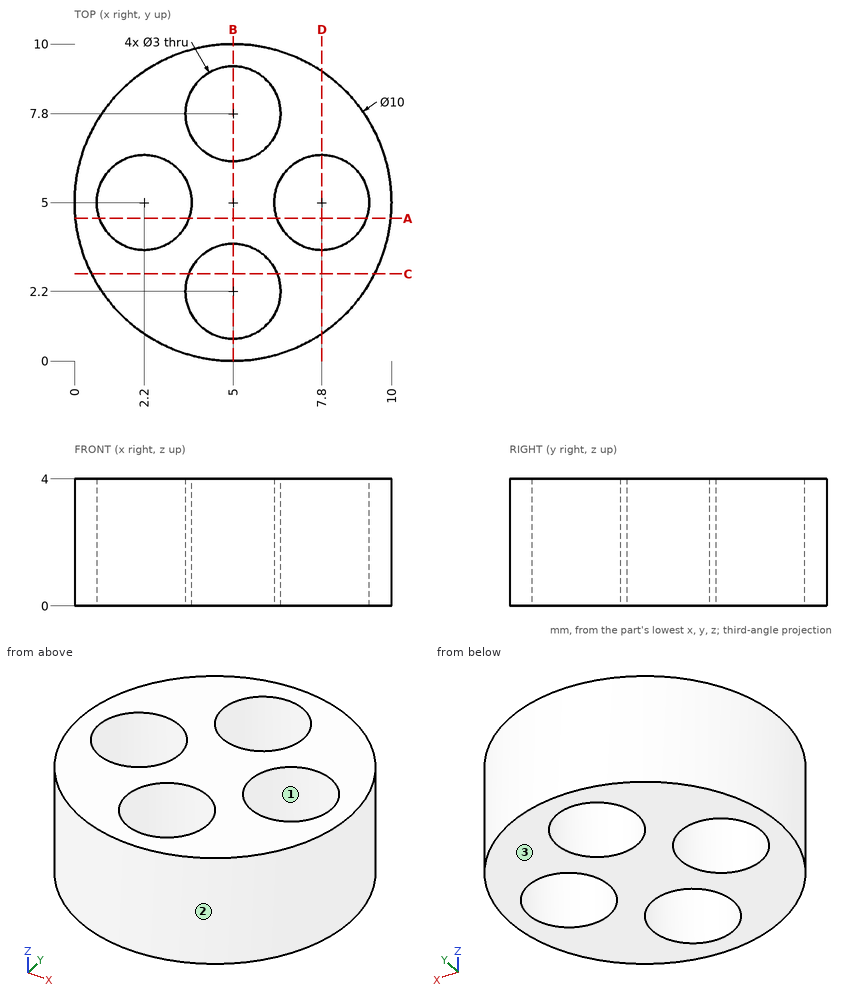
For this review, use the dimensioned drawing (mm, ordinates from the lowest corner) and the shaded views. Coordinates: 2 decimals unless noted, no trailing zeros. Order: outer loops, then holes, each group sorted by start corner. A loop starts at its lowest first (then second) coordinate and runs counter-clockwise, first axis right, second up. Notation, with made-up numbers: (75.25, 42.25) - (116.25, 42.25) arc R9 ccw to (116.25, 54.25) - close; hole circle Ø9 at (22, 51.5). An arc over 180 degrees is marked (long way). Answer as a JSON object with one key per item and string values. Group by question number.
1. We need section D-D on x = 7.8. State the section outline as (y, z) points.
2. We need section C-C on y = 2.75. State the section outline as (x, z) points, then the cut area to 3 significant figures.
3. For probe 1 along X at (y, z) = (5, 3.6); probe 2 along Y at (x, z) = (6.25, 2); probe 3 along X at (y, z) = (1, 3.5), list the stretches that pass through material, from the lowest coordinate up.
4. Clearance check with flat-ended pins moving along their axes: P1, Ø1.5, axis at y = 6, z = 3.5, coming from the -X side; P2, Ø2.5, axis at x = 7.8, y = 5, coming from the +Z side; P3, Ø1.5, axis at y = 7, z = 3.5, coming from the +X side. State where each tip first meets the part, or that it passes through.
5. We need section A-A on y = 4.5. State the section outline as (x, z) points.
6. We need section B-B on x = 5. State the section outline as (y, z) points.
7. The part is to be moulded in two halves that separate along Y. For the marked faces 1, 2 and 3, say which applies: pulls with the +Y half, pulls with the -Y half, needs draft (parallel to the pull), parting line crosses it, or undercut.
Final values:
{
 "1": {"outline": "(0.86, 0) - (3.5, 0) - (3.5, 4) - (0.86, 4) - close; (6.5, 0) - (9.14, 0) - (9.14, 4) - (6.5, 4) - close"},
 "2": {"outline": "(0.53, 0) - (3.6, 0) - (3.6, 4) - (0.53, 4) - close; (6.4, 0) - (9.47, 0) - (9.47, 4) - (6.4, 4) - close", "area": "24.6 mm²"},
 "3": {"probe 1": "0 to 0.7, 3.7 to 6.3, 9.3 to 10", "probe 2": "0.16 to 1.37, 3.03 to 6.97, 8.63 to 9.84", "probe 3": "2 to 4.1, 5.9 to 8"},
 "4": {"P1": "x = 0.01", "P2": "through", "P3": "x = 9.84"},
 "5": {"outline": "(0.03, 0) - (0.79, 0) - (0.79, 4) - (0.03, 4) - close; (3.61, 0) - (6.39, 0) - (6.39, 4) - (3.61, 4) - close; (9.21, 0) - (9.97, 0) - (9.97, 4) - (9.21, 4) - close"},
 "6": {"outline": "(0, 0) - (0.7, 0) - (0.7, 4) - (0, 4) - close; (3.7, 0) - (6.3, 0) - (6.3, 4) - (3.7, 4) - close; (9.3, 0) - (10, 0) - (10, 4) - (9.3, 4) - close"},
 "7": {"face 1": "undercut", "face 2": "parting line crosses it", "face 3": "needs draft"}
}
